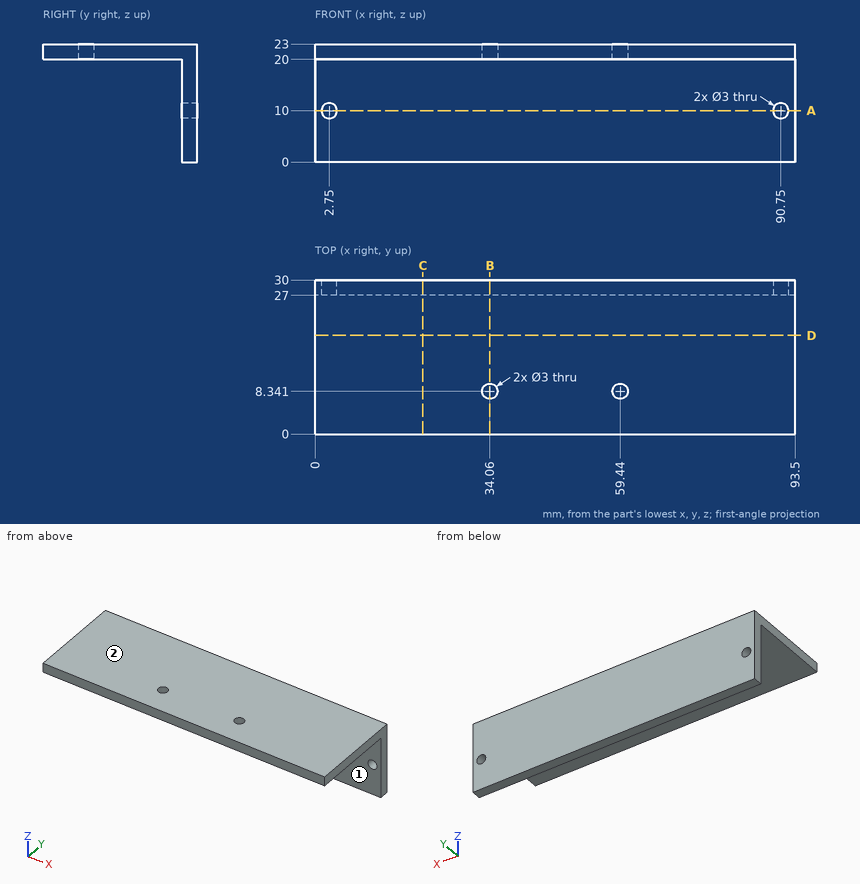
The figure shows three views and two pictorial views of one solid part (mm, origin at its lowest corner). Answer the questions. A direction names the side the tool comes from. Coordinates: 2 decimals unless noted, no trailing zeros. Loops run counter-clockwise (first coordinate to the right, second up) from the corner with the lowest first, then second, coordinate; pieces in that order, holes last. Notation, with made-up numbers: (-27.5, 71.5) - (-18.5, 71.5) arc R15 ccw to (-18.5, 83.5) - close; hole circle Ø3 at (-14.5, 67). An arc over 180 degrees is marked (long way). Answer in a Markdown table with one row per item.
Q1. Find section C-C on x = 21. Write down the section's boundary in (y, z).
Here are the results:
| item | result |
|---|---|
| outline | (0, 20) - (27, 20) - (27, 0) - (30, 0) - (30, 23) - (0, 23) - close |
Q2. Given P1, Ø3, axis at x = 71, z = 15, coming from the -Y side; P2, Ø13.5, axis at x = 53, y = 18, coming from the -Z side; P3, Ø2.5, axis at x = 90.75, z = 10, coming from the -Y side, each flat-ended and moving along its own axis, determine where each tip first touches the part or whether it passes through.
Here are the results:
| item | result |
|---|---|
| P1 | stops at y = 27 |
| P2 | stops at z = 20 |
| P3 | passes through |
Q3. Find section A-A on z = 10. Write down the section's boundary in (x, y).
Here are the results:
| item | result |
|---|---|
| outline | (0, 27) - (1.25, 27) - (1.25, 30) - (0, 30) - close; (4.25, 27) - (89.25, 27) - (89.25, 30) - (4.25, 30) - close; (92.25, 27) - (93.5, 27) - (93.5, 30) - (92.25, 30) - close |
Q4. Find section D-D on y = 19.25. Write down the section's boundary in (x, z).
Here are the results:
| item | result |
|---|---|
| outline | (0, 20) - (93.5, 20) - (93.5, 23) - (0, 23) - close |
Q5. Find section B-B on x = 34.06. Write down the section's boundary in (y, z), plus the area to 3 significant figures.
Here are the results:
| item | result |
|---|---|
| outline | (0, 20) - (6.84, 20) - (6.84, 23) - (0, 23) - close; (9.84, 20) - (27, 20) - (27, 0) - (30, 0) - (30, 23) - (9.84, 23) - close |
| area | 141 mm^2 |
Q6. For the marked faces 1 and 2, determine the directions among +Z, -Z, +X, -X, +Y, -Y from which every point of the face is accessible in a straight line to the end or side of a thin tool.
Here are the results:
| item | result |
|---|---|
| face 1 | -Z, +X, -X, -Y |
| face 2 | +Z, +X, -X, +Y, -Y |
Q7. Straight lines are drawn through the part: line 1 along Y through (x, z) = (34.06, 22.05); line 2 along Z through (x, y) = (2.75, 28.5); line 3 along Y through (x, z) = (76, 5). For each, find the intervals that lie inside material, in ascending order. Write a range as [from, to].
Here are the results:
| item | result |
|---|---|
| line 1 | y = [0, 6.84], [9.84, 30] |
| line 2 | z = [0, 8.5], [11.5, 23] |
| line 3 | y = [27, 30] |
